CAD build for the part. Positions are in the model's coordinates, mm. A direction names the side the tool comes from. Coordinates: 2 decimals unless noted, no trailing zeros. Loops run counter-clockwise (first coordinate to the right, second up) from the corner with the lowest first, then second, coordinate; pieces in that order, holes last.
1) Two-plate mould, pull along Z, no slides. Class faces 4 (the flat face through (5, 4, 0)), 5 (the cylindrical face through (3.52, -3.16, 2.02)), 6 (the cylindrical face through (-4.493, -6.083, -6.633)): +Z half, -Z half, draft (parallel to the pull), parting line (faces both ways), or undercut.
2) Saw through at B-B, the plane x = -0.25. Write the cut outline in (y, z), and give its area (3 significant figures).
3) Wall check: line 1 along X through (y, z) = (-2.75, 0); line 2 along Y through (x, z) = (3.35, 0); line 3 along Z through (x, y) = (3.5, -3). Give the ranges that are in metal, low to high.
4) Which spindle directions (+Z, -Z, +X, -X, +Y, -Y) get a long thin tool onto all of the face, cutting with end or side? Do faces 1 (the flat face through (2, 2, -2)), 2 (the flat face through (-5, 4, 0)), 3 (the cylindrical face through (-3.52, -3.16, 2.02)). Say none if no direction does.
5) Pin check, flat tips, straight feed: pin 1 Ø2 at (y, z) = (-1.5, 1.5) entering from -X; pin 2 Ø6 at (y, z) = (1, 0) entering from +X; pin 3 Ø6 at (x, y) = (-1.5, 6.5) entering from -Z; pin 4 Ø2 at (x, y) = (-0.5, -1.5) entering from -Z. Stop position of each tip, or through.
6) Saw through at A-A, the plane x = -3.5. Write the cut outline in (y, z).
```python
from build123d import *
from build123d.topology import SkipClean


with BuildPart() as part:
    # Sketch1 → Revolve1 (revolve)
    with BuildSketch(Plane.XY, mode=Mode.PRIVATE) as revolve1_sk:
        with BuildLine():
            Line((0, 2), (2, 2))
            Line((2, 2), (2, 3.75))
            Line((2, 3.75), (5, 3.75))
            Line((5, 3.75), (5, 9))
            Line((5, 9), (4, 9))
            ThreePointArc((4, 9), (2.236067977, 7.527864045), (0, 7))
            Line((0, 7), (0, 2))
        make_face()
    revolve1 = revolve(revolve1_sk.sketch.rotate(Axis((0, 0, 0), (1, 0, 0)), 90), axis=Axis((0, 0, 0), (1, 0, 0)))

    # Mirror1: Revolve1 across plane
    with SkipClean():  # the faces are left unmerged after this step: merging them gives an invalid solid
        add(revolve1.mirror(Plane(origin=(0, 2, 0), x_dir=(0, 0, 1), z_dir=(1, 0, 0))))


solid = part.part
```
Data:
1. face 4: draft
1. face 5: undercut
1. face 6: parting line
2. outline: circle Ø14.01 at (0, 0); hole circle Ø4 at (0, 0)
2. area: 142 mm2
3. line 1: x = -2 to 2
3. line 2: y = -8.29 to -3.75, 3.75 to 8.29
3. line 3: z = -7.88 to -2.25, 2.25 to 7.88
4. face 1: +X
4. face 2: +Z, -Z, -X, +Y, -Y
4. face 3: -X
5. pin 1: stops at x = -2
5. pin 2: stops at x = 5
5. pin 3: stops at z = -7.59
5. pin 4: stops at z = -7.12
6. outline: circle Ø16.86 at (0, 0); hole circle Ø7.5 at (0, 0)
